Check sheet for the modelled part. Datum: model origin and axes. Units: mm. Face numbers are marked on the shaded views. A direction names the side the tool comes from. Give positions to 0.01 mm unless a question says otherwise; leave off trailing zeros. Order: outer loops, then holes, each group sorted by start corner. A loop starts at its lowest first (then second) coordinate and runs counter-clockwise, first axis right, second up.
from build123d import *

# Parameters (mm, degrees)
F1_DEPTH  = 15.875
F2_R      = 3.96875
F3_DEPTH  = 127
F5_DEPTH  = 15.876
F7_DEPTH  = 25.4
F8_R      = 3.96875
F9_DEPTH  = 25.4
F10_W     = 12.7
F10_H     = 25.4
F11_DEPTH = 3.175


with BuildPart() as f1:
    # F0 (on Top) → F1 (new body)
    with BuildSketch(Plane.XY):
        Polygon((-101.6, 63.5), (-114.3, 50.8), (-114.3, -50.8), (-101.6, -63.5), (114.3, -63.5), (114.3, 63.5), align=None)
    extrude(amount=F1_DEPTH)

    # F2 (on Front) → F3 (cut, symmetric)
    with BuildSketch(Plane.XZ):
        with Locations((-76.2, 7.9375)):
            Circle(F2_R)
        with Locations((88.9, 7.9375)):
            Circle(F2_R)
    extrude(amount=F3_DEPTH, both=True, mode=Mode.SUBTRACT)

    # F4 (on face) → F5 (cut, through all)
    with BuildSketch(Plane.XY.offset(15.875)):
        Polygon((76.2, 50.8), (38.1, 12.7), (38.1, -12.7), (76.2, -50.8), (101.6, -50.8), (101.6, 50.8), align=None)
    extrude(amount=-F5_DEPTH, mode=Mode.SUBTRACT)

    # F6 (on face) → F7 (cut)
    with BuildSketch(Plane.XY.offset(15.875)):
        Polygon((-38.1, -12.7), (-38.1, 12.7), (-63.5, 50.8), (-88.9, 50.8), (-101.6, 38.1), (-101.6, -38.1), (-88.9, -50.8), (-63.5, -50.8), align=None)
    extrude(amount=-F7_DEPTH, mode=Mode.SUBTRACT)

    # F8 (on face) → F9 (join)
    with BuildSketch(Plane.XY.offset(15.875)):
        Circle(F8_R)
    extrude(amount=F9_DEPTH)

    # F10 (on face) → F11 (join)
    with BuildSketch(Plane.XY.offset(15.875)):
        with Locations((-76.2, 57.15)):
            Rectangle(F10_W, F10_H)
        with Locations((-76.2, -57.15)):
            Rectangle(F10_W, F10_H)
    extrude(amount=F11_DEPTH)


solid = f1.part
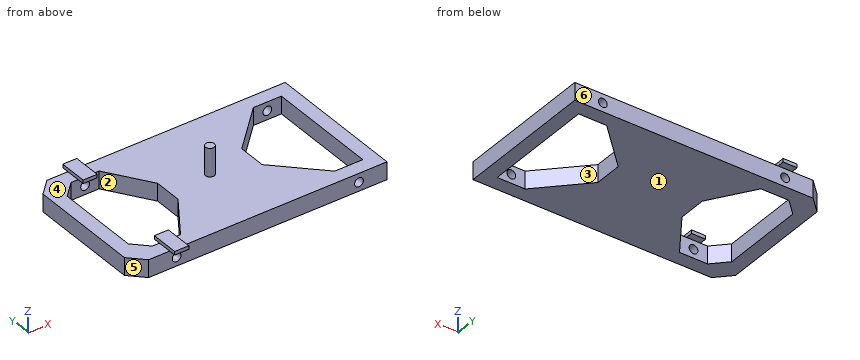
1) Depth check by flat-ended pin: pin 1 Ø8 at (x, z) = (44, 7) entering from +Y; pin 2 Ø17.5 at (x, z) = (21, 6) entering from -Y; pin 3 Ø6.5 at (x, y) = (-76.5, -53.5) entering from +Z. Enter the tip coordinate at first touch or a pass-through.
Recorded:
pin 1: stops at y = 63.5
pin 2: stops at y = -63.5
pin 3: stops at z = 19.05
2) Set-up check for the marked faces 1 and 2: record each of +Z, -Z, +X, -X, +Y, -Y from which the full face is reachable in a straight line by a thin tool's end or side.
Recorded:
face 1: -Z, +X, -X, +Y, -Y
face 2: +Z, -Z
3) Draft check along Y on the marked faces 3, 4, 5 and 6. Enter one of: +Y half, -Y half, draft (parallel to the pull), parting line (faces both ways), or undercut.
Recorded:
face 3: undercut
face 4: draft
face 5: -Y half
face 6: +Y half
4) Section check B-B, the plane y = -8. Record the cut outline in (x, z) (3 decimals).
Recorded:
outline: (-114.3, 0) - (-101.6, 0) - (-101.6, 15.875) - (-114.3, 15.875) - close; (-38.1, 0) - (38.1, 0) - (38.1, 15.875) - (-38.1, 15.875) - close; (101.6, 0) - (114.3, 0) - (114.3, 15.875) - (101.6, 15.875) - close
5) Material ranges on L1, parallel to X at y = 1, z = 11; L2, parallel to X at y = -26, z = 6.5; L3, parallel to Z at x = -76, y = -53, recorded low to high.
Recorded:
L1: x = -114.3 to -101.6, -38.1 to 38.1, 101.6 to 114.3
L2: x = -114.3 to -101.6, -46.97 to 51.4, 101.6 to 114.3
L3: z = 0 to 3.97, 11.9 to 19.05
6) Section check C-C, the plane x = 88.9. Record the cut outline in (y, z) (3 decimals).
Recorded:
outline: (-63.5, 0) - (-50.8, 0) - (-50.8, 3.969) - (-63.5, 3.969) - close; (-63.5, 11.906) - (-50.8, 11.906) - (-50.8, 15.875) - (-63.5, 15.875) - close; (50.8, 0) - (63.5, 0) - (63.5, 3.969) - (50.8, 3.969) - close; (50.8, 11.906) - (63.5, 11.906) - (63.5, 15.875) - (50.8, 15.875) - close
7) Section check A-A, the plane x = 48. Record the cut outline in (y, z) (3 decimals).
Recorded:
outline: (-63.5, 0) - (-22.6, 0) - (-22.6, 15.875) - (-63.5, 15.875) - close; (22.6, 0) - (63.5, 0) - (63.5, 15.875) - (22.6, 15.875) - close
8) Section check D-D, the plane x = 0. Record the cut outline in (y, z) (3 decimals), then the cut area to 3 significant figures.
Recorded:
outline: (-63.5, 0) - (63.5, 0) - (63.5, 15.875) - (3.969, 15.875) - (3.969, 41.275) - (-3.969, 41.275) - (-3.969, 15.875) - (-63.5, 15.875) - close
area: 2,220 mm2
